Geometry check sheet. Reference: drawing and pictorial views, mm from the part's lowest x, y, z. A direction names the side the tool comes from. Give positions to 0.01 mm unless a question says otherwise; leave off trailing zeros. Write each loop counter-clockwise with the first axis right and the second up, starting at its lowest first coordinate (ties: lowest second). Pieces come first, ordered by that corner, then holes. Notation, with made-up numbers: (8, 81.5) -> (55, 81.5) arc R13 ccw to (55, 106.5) -> close; hole circle Ø1 at (50.25, 31). An arc over 180 degrees is marked (long way). Return JSON: item names as keys, results as strings.
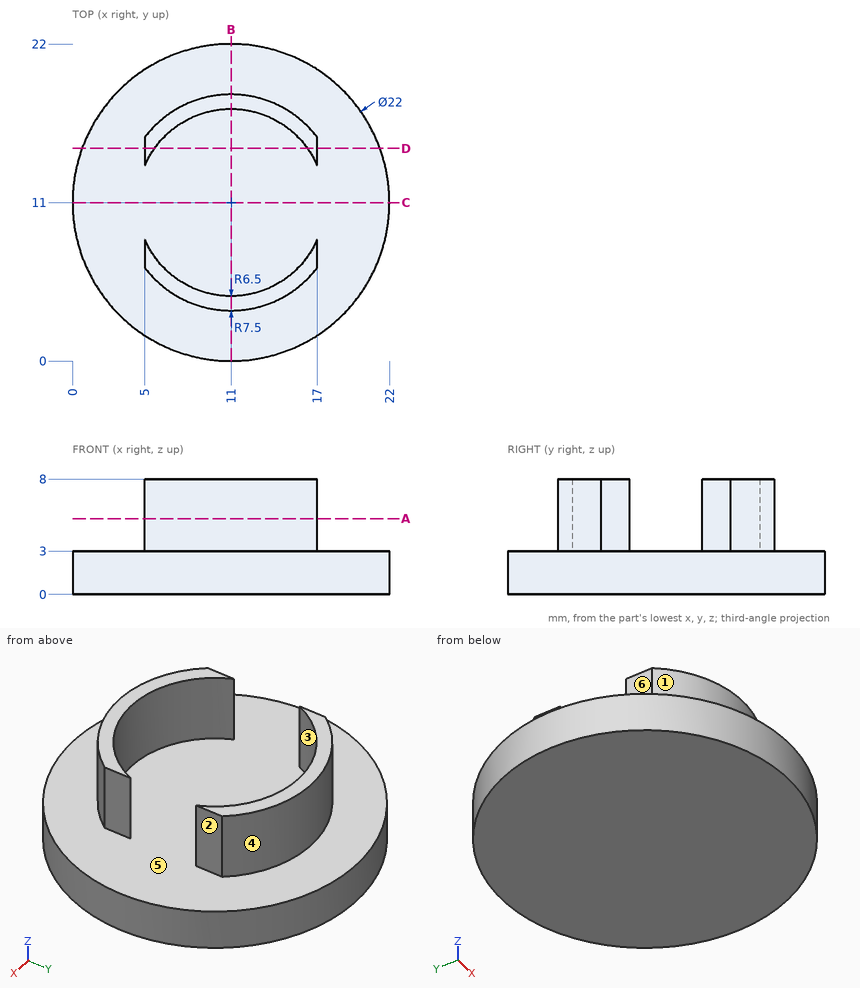
(1) Cross-section at D-D on y = 14.75. Enter the section's corners in (x, z).
Reply:
{"outline": "(0.66, 0) -> (21.34, 0) -> (21.34, 3) -> (17, 3) -> (17, 8) -> (16.31, 8) -> (16.31, 3) -> (5.69, 3) -> (5.69, 8) -> (5, 8) -> (5, 3) -> (0.66, 3) -> close"}
(2) Cross-section at B-B on x = 11. Enter the section's corners in (y, z), then the cut area to 3 significant figures.
Reply:
{"outline": "(0, 0) -> (22, 0) -> (22, 3) -> (18.5, 3) -> (18.5, 8) -> (17.5, 8) -> (17.5, 3) -> (4.5, 3) -> (4.5, 8) -> (3.5, 8) -> (3.5, 3) -> (0, 3) -> close", "area": "76.0 mm^2"}
(3) Depth check by flat-ended pin: pin 1 Ø1.6 at (y, z) = (14.5, 4.5) entering from +X; pin 2 Ø0.6 at (y, z) = (15, 5) entering from -X; pin 3 Ø4 at (x, z) = (17, 1) entering from -Y. Enter the tip coordinate at first touch or a pass-through.
Reply:
{"pin 1": "x = 17", "pin 2": "x = 5", "pin 3": "y = 0.75"}
(4) Thickness scan on L1, parallel to X at y = 6.75, z = 3.25; L2, parallel to Z at x = 3, y = 12.5; L3, parallel to X at y = 6, z = 5. Record the ranges inside material, lowest first.
Reply:
{"L1": "5 to 6.08, 15.92 to 17", "L2": "0 to 3", "L3": "5.41 to 6.85, 15.15 to 16.59"}
(5) Cross-section at C-C on y = 11. Enter the section's corners in (x, z), then the cut area to 3 significant figures.
Reply:
{"outline": "(0, 0) -> (22, 0) -> (22, 3) -> (0, 3) -> close", "area": "66.0 mm^2"}
(6) Set-up check for the marked faces 1, 2 and 3: record each of +Z, -Z, +X, -X, +Y, -Y from which the full face is reachable in a straight line by a thin tool's end or side.
Reply:
{"face 1": "+Z, -Y", "face 2": "+Z, +X, +Y, -Y", "face 3": "+Z"}
(7) Cross-section at A-A on z = 5.25. Enter the section's corners in (x, y).
Reply:
{"outline": "(5, 6.5) arc R7.5 ccw to (17, 6.5) -> (17, 8.5) arc R6.5 cw to (5, 8.5) -> close; (5, 13.5) arc R6.5 cw to (17, 13.5) -> (17, 15.5) arc R7.5 ccw to (5, 15.5) -> close"}
(8) Release check for a two-part mould opening along X. For the marked faces 4, 5 and 6 record: pulls with the +X half, pulls with the -X half, needs draft (parallel to the pull), parting line crosses it, or undercut.
Reply:
{"face 4": "parting line crosses it", "face 5": "undercut", "face 6": "pulls with the -X half"}
